Input: part model. Units: mm. Frame: model coordinates. Give positions to 0.01 mm unless a question says otherwise; leave off trailing zeros. Loops run counter-clockwise (first coordinate to the right, second up) from the corner with the lowest first, then second, coordinate; pieces in that order, holes last. Notation, with made-up numbers: M 23,-19.5 L 27,-19.5 A20 cw 27,12.5 Z; hole C -37.75,-4.75 d3. An arc over 180 degrees is marked long. One line per item, written item: value. Start each with the question number.
(1) Section A-A on z = 16. Output: boundary loops of the cut face in (x, y), plus the area to 3 significant figures.
(2) Ray query, line 1 along X through (y, z) = (6.5, 17); line 2 along X through (y, z) = (3.5, 11). Return the intervals inside material, ascending. Write a range as from..to.
(3) Pin query (flat end, axial travel): P1, Ø2, axis at y = 5, z = 15, coming from the +X side; P2, Ø5, axis at x = 13.5, z = 7, coming from the -Y side. Return the tip coordinate at first contact, or that it passes through.
```python
from build123d import *

# Parameters (mm, degrees)
EXTRUDE_1_DEPTH = 8


with BuildPart() as part:
    # Эскиз1 → Бобышка-Вытянуть1 (new body)
    with BuildSketch(Plane(origin=(0, 0, 0), x_dir=(1, 0, 0), z_dir=(0, 1, 0))):
        with BuildLine():
            Line((-25, -20), (15, -20))
            ThreePointArc((15, -20), (22.071067812, -17.071067812), (25, -10))
            Line((25, -10), (25, 20))
            Line((25, 20), (-25, 20))
            Line((-25, 20), (-25, -20))
        make_face()
    extrude(amount=EXTRUDE_1_DEPTH)


solid = part.part
```
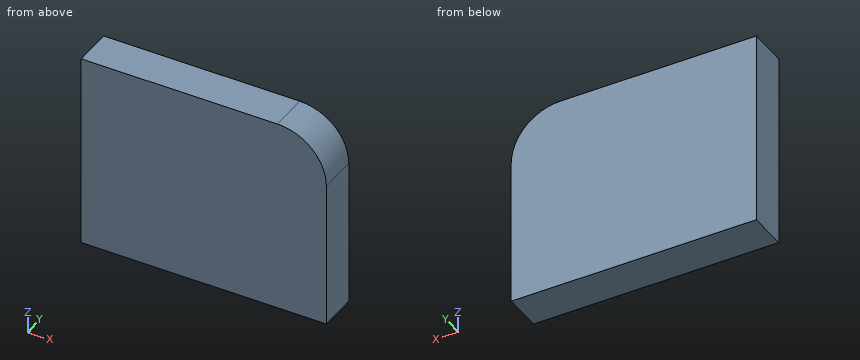
Output values:
1. outline: M -25,0 L 23,0 L 23,8 L -25,8 Z
1. area: 384 mm²
2. line 1: x = -25..22.14
2. line 2: x = -25..24.95
3. P1: stops at x = 24.17
3. P2: stops at y = 0
